Input: part model. Units: mm. Frame: model coordinates. A direction names the side the tool comes from. Give positions to 0.01 mm unless a question says otherwise; leave off trailing zeros. Loops run counter-clockwise (first coordinate to the right, second up) from the corner with the lowest first, then second, coordinate; pieces in that order, holes last. Notation, with made-up numbers: (59.25, 30.5) -> (85.25, 30.5) arc R7 cw to (85.25, 34.5) -> close; hole circle Ø7 at (-7.5, 29). An arc over 180 degrees is marked (long way). Answer as a JSON object with one key per item and string values. Group by question number.
Autodesk Inventor part; units mm, degrees
ref_plane "YZ Plane" through (0, 0, 0) normal (1, 0, 0) x (0, 1, 0)
ref_plane "XZ Plane" through (0, 0, 0) normal (0, 1, 0) x (-1, 0, 0)
ref_plane "XY Plane" through (0, 0, 0) normal (0, 0, 1) x (1, 0, 0)
sketch "Sketch1" plane through (0, 0, 0) normal (1, 0, 0) x (0, 1, 0)
  line L0 (0, 0) -> (0, -110)
  line L1 (0, 0) -> (110, 0) construction
  line L2 (0, -110) -> (70, -110)
  line L3 (0, -110) -> (70, -110) construction
  line L4 (70, -110) -> (70, -130)
  line L5 (70, -130) -> (155, -130)
  line L6 (70, -130) -> (155, -130) construction
  line L7 (155, -130) -> (155, -110)
  line L8 (155, -110) -> (85, -110)
  line L9 (85, -110) -> (85, 0)
  line L10 (85, 0) -> (155, 0)
  line L11 (155, 0) -> (155, 20)
  line L12 (155, 20) -> (70, 20)
  line L13 (70, 20) -> (70, 0)
  line L14 (70, 0) -> (0, 0)
  dimension "d0" = 110
  dimension "d1" = 90
  dimension "d2" = 70
  dimension "d3" = 0
  dimension "d4" = 20
  dimension "d5" = 85
  dimension "d6" = 0
  dimension "d7" = 20
  dimension "d8" = 70
  dimension "d9" = 110
  dimension "d10" = 90
  dimension "d11" = 70
  dimension "d12" = 90
  dimension "d13" = 20
  dimension "d14" = 90
  dimension "d15" = 85
  dimension "d16" = 90
extrude "Extrusion1" add sketch "Sketch1" along normal blind 5
sketch "Sketch2" plane through (5, 0, 0) normal (1, 0, 0) x (0, 0, -1)
  point P0 (0, 0)
  point P1 (55, 40)
sketch "Sketch3" plane through (5, 0, 0) normal (1, 0, 0) x (0, 0, -1)
  circle A0 centre (55, 40) radius 1.5
  point P0 (0, 0)
  dimension "d19" = 3
extrude "Extrusion2" add sketch "Sketch3" along normal blind 30
sketch "Sketch4" plane through (0, 0, 0) normal (-1, 0, 0) x (0, 0, 1)
  line L0 (-67, 42.5) -> (-43, 42.5)
  line L1 (-43, 42.5) -> (-43, 37.5)
  line L2 (-43, 37.5) -> (-67, 37.5)
  line L3 (-67, 37.5) -> (-67, 42.5)
  circle A0 centre (-55, 40) radius 1.5
  line L4 (-67, 42.5) -> (-43, 37.5) construction
  line L5 (-43, 42.5) -> (-67, 37.5) construction
  point P0 (0, 0)
  dimension "d22" = 24
  dimension "d23" = 5
sketch "Sketch5" plane through (0, 0, 0) normal (-1, 0, 0) x (0, 0, 1)
  point P0 (0, 0)
sketch "Sketch6" plane through (0, 0, 0) normal (-1, 0, 0) x (0, 0, 1)
  circle A0 centre (-55, 40) radius 1.5
  point P0 (0, 0)
extrude "Extrusion3" add sketch "Sketch4" along normal blind 20 contours L0 L1 L2 L3 | A0
sketch "Sketch7" plane through (0, 42.5, -43) normal (0, 1, 0) x (1, 0, 0)
  line L0 (-20, 24) -> (-20, 0)
  line L1 (0, 24) -> (-20, 24)
  line L2 (-20, 0) -> (-15, 0)
  line L3 (-15, 0) -> (-15, 24)
  line L4 (-15, 24) -> (-20, 24)
  line L5 (-20, 24) -> (-20, 0)
  point P0 (0, -43)
  dimension "d26" = 5
extrude "Extrusion4" add sketch "Sketch7" along normal blind 45
sketch "Sketch9" plane through (5, 0, 0) normal (1, 0, 0) x (0, 0, -1)
  point P0 (0, 0)
properties part number "part1 edited" material "Wood (Walnut)"
Q1. Set-up query: faces 1 (the face through (2, 120, -110)), 2 (the face through (-16, 57, -67)), 3 (the face through (2, 70, -120)). Return all of +Z, -Z, +X, -X, +Y, -Y with unobstructed straight access to the full face (end or side cutting, diameter ignored); none if empty.
Q2. Section D-D on x = -4. Return the cut outline in (y, z).
Q3. Pin query (flat end, axial travel): pin 1 Ø12 at (x, z) = (-8.5, -59) entering from +Y; pin 2 Ø8 at (x, z) = (29, -49) entering from -Y; pin 3 Ø4 at (x, z) = (6.5, -110.5) entering from -Y; pin 4 Ø4 at (x, y) = (3, 27) entering from +Z. Return the tip coordinate at first contact, or that it passes through.
Q4. Ray query, probe 1 along X at (y, z) = (82.5, -59.5); probe 2 along X at (y, z) = (31.5, -6.5); probe 3 along Y at (x, z) = (-1.5, -48). Return the intervals inside material, ascending.
Q5. Section B-B on z = -3.5. Return the cut outline in (x, y).
Q6. Pull-direction query (X, two-part tool) for faces 4 (the face through (-20, 62, -55)), 5 (the face through (2, 112, -130)), 6 (the face through (-15, 65, -55)); classes: +X half, -X half, draft (parallel to the pull), parting line (faces both ways), or undercut.
Q7. Section C-C on y = 56.5. Return the cut outline in (x, z), then the cut area to 3 significant figures.
Q8. Section A-A on y = 145. Return the cut outline in (x, z).
Numbers:
{
 "1": {"face 1": "+X, -X, +Y", "face 2": "-Z, -X, +Y, -Y", "face 3": "-Z, +X, -X, -Y"},
 "2": {"outline": "(37.5, -67) -> (42.5, -67) -> (42.5, -43) -> (37.5, -43) -> close"},
 "3": {"pin 1": "stops at y = 42.5", "pin 2": "passes through", "pin 3": "stops at y = 0", "pin 4": "stops at z = 0"},
 "4": {"probe 1": "x = -20 to -15, 0 to 5", "probe 2": "x = 0 to 5", "probe 3": "y = 37.5 to 42.5"},
 "5": {"outline": "(0, 0) -> (5, 0) -> (5, 85) -> (0, 85) -> close"},
 "6": {"face 4": "-X half", "face 5": "draft", "face 6": "undercut"},
 "7": {"outline": "(-20, -67) -> (-15, -67) -> (-15, -43) -> (-20, -43) -> close; (0, -110) -> (5, -110) -> (5, 0) -> (0, 0) -> close", "area": "670 mm²"},
 "8": {"outline": "(0, -130) -> (5, -130) -> (5, -110) -> (0, -110) -> close; (0, 0) -> (5, 0) -> (5, 20) -> (0, 20) -> close"}
}
